```python
from build123d import *

# Parameters (mm, degrees)
SKETCH1_W           = 42
SKETCH1_H           = 42
BOSS_EXTRUDE1_DEPTH = 2
CUT_EXTRUDE1_DEPTH  = 10
SKETCH3_R           = 5
CUT_EXTRUDE2_DEPTH  = 10
SKETCH4_R           = 2
CUT_EXTRUDE3_DEPTH  = 10
SKETCH5_W           = 7
SKETCH5_H           = 10
CUT_EXTRUDE4_DEPTH  = 4


with BuildPart() as part:
    # Sketch1 → Boss-Extrude1 (new body)
    with BuildSketch(Plane(origin=(0, 0, 0), x_dir=(1, 0, 0), z_dir=(0, 1, 0))):
        Rectangle(SKETCH1_W, SKETCH1_H)
    extrude(amount=BOSS_EXTRUDE1_DEPTH)

    # Sketch2 → Cut-Extrude1 (cut)
    with BuildSketch(Plane(origin=(0, 2, 0), x_dir=(1, 0, 0), z_dir=(0, 1, 0))):
        Polygon((-16.050252532, 21), (-21, 21), (-21, 16.050252532), align=None)
        Polygon((21, 21), (16.050252532, 21), (21, 16.050252532), align=None)
        Polygon((21, -16.050252532), (16.050252532, -21), (21, -21), align=None)
        Polygon((-16.050252532, -21), (-21, -16.050252532), (-21, -21), align=None)
    extrude(amount=-CUT_EXTRUDE1_DEPTH, mode=Mode.SUBTRACT)

    # Sketch3 → Cut-Extrude2 (cut)
    with BuildSketch(Plane(origin=(0, 2, 0), x_dir=(1, 0, 0), z_dir=(0, 1, 0))):
        with Locations(Location((0, 0, 0), (0, 0, 270))):
            Circle(SKETCH3_R)
    extrude(amount=-CUT_EXTRUDE2_DEPTH, mode=Mode.SUBTRACT)

    # Sketch4 → Cut-Extrude3 (cut)
    with BuildSketch(Plane.XZ):
        with Locations(Location((6.5, 15.5, 0), (0, 0, 270))):
            Circle(SKETCH4_R)
        with Locations(Location((-6.5, -15.5, 0), (0, 0, 270))):
            Circle(SKETCH4_R)
    extrude(amount=-CUT_EXTRUDE3_DEPTH, mode=Mode.SUBTRACT)

    # Sketch5 → Cut-Extrude4 (cut)
    with BuildSketch(Plane.XZ):
        with Locations((0, -16)):
            Rectangle(SKETCH5_W, SKETCH5_H)
        with Locations((0, 16)):
            Rectangle(SKETCH5_W, SKETCH5_H)
    extrude(amount=-CUT_EXTRUDE4_DEPTH, mode=Mode.SUBTRACT)


solid = part.part
```
For this review, take the finished solid that the model builds, in its own axes (mm). A direction names the side the tool comes from. Round coordinates to 2 decimals unless told otherwise and drop trailing zeros. Loops run counter-clockwise (first coordinate to the right, second up) from the corner with the lowest first, then second, coordinate; pieces in that order, holes last.
Q1. Add section D-D on z = 15.5. Write out the cut boundary in (x, y).
Result sheet:
outline: (-21, 0) - (-3.5, 0) - (-3.5, 2) - (-21, 2) - close; (3.5, 0) - (4.5, 0) - (4.5, 2) - (3.5, 2) - close; (8.5, 0) - (21, 0) - (21, 2) - (8.5, 2) - close
Q2. Add section C-C on y = 1.15. Write out the cut boundary in (x, z).
Result sheet:
outline: (-21, -16.05) - (-16.05, -21) - (-3.5, -21) - (-3.5, -11) - (3.5, -11) - (3.5, -21) - (16.05, -21) - (21, -16.05) - (21, 16.05) - (16.05, 21) - (3.5, 21) - (3.5, 11) - (-3.5, 11) - (-3.5, 21) - (-16.05, 21) - (-21, 16.05) - close; hole circle Ø4 at (-6.5, -15.5); hole circle Ø10 at (0, 0); hole circle Ø4 at (6.5, 15.5)
Q3. Mouldability with a two-part tool opening along Z and no side actions: class faces 1 (the face through (4, 2, 4)), 2 (the face through (-10, 1, -21)), 3 (the face through (-4.88, 1.01, -1.08)) as +Z half, -Z half, draft (parallel to the pull), parting line (faces both ways), or undercut.
Result sheet:
face 1: draft
face 2: -Z half
face 3: undercut
Q4. Machinability: for faces 4 (the face through (3.5, 1, 16)), 5 (the face through (18.49, 1.01, -18.56)), 6 (the face through (-3.5, 1, -16)), which of the approach directions +Z, -Z, +X, -X, +Y, -Y give a long, thin tool a straight path to every point of the face, cutting with its end or side? Answer none if there is none.
Result sheet:
face 4: +Z, +Y, -Y
face 5: -Z, +X, +Y, -Y
face 6: -Z, +Y, -Y
Q5. To check wall thickness, follow line 1 along X through (y, z) = (1.15, -15.5); line 2 along X through (y, z) = (0.55, 15.5); line 3 along X through (y, z) = (0.8, -12). State the ranges of each line that lie inside material, in increasing order.
Result sheet:
line 1: x = -21 to -8.5, -4.5 to -3.5, 3.5 to 21
line 2: x = -21 to -3.5, 3.5 to 4.5, 8.5 to 21
line 3: x = -21 to -3.5, 3.5 to 21
Q6. Insertion check: pin 1 Ø0.6 at (x, y) = (1.5, 1) entering from +Z; pin 2 Ø1 at (x, y) = (1, 1.5) entering from -Z; pin 3 Ø2.5 at (x, z) = (-6.5, -15.5) entering from +Y; pin 4 Ø0.6 at (y, z) = (1, -18) entering from +X. Each pin has a flat end and moves straight along its axis. Give the tip position at first contact, or say it passes through.
Result sheet:
pin 1: stops at z = 11
pin 2: stops at z = -11
pin 3: passes through
pin 4: stops at x = 19.35
Q7. Add section A-A on x = 0. Write out the cut boundary in (y, z), plus the area to 3 significant figures.
Result sheet:
outline: (0, -11) - (2, -11) - (2, -5) - (0, -5) - close; (0, 5) - (2, 5) - (2, 11) - (0, 11) - close
area: 24.0 mm2
Q8. Add section B-B on z = 0. Write out the cut boundary in (x, y), plus the area to 3 significant figures.
Result sheet:
outline: (-21, 0) - (-5, 0) - (-5, 2) - (-21, 2) - close; (5, 0) - (21, 0) - (21, 2) - (5, 2) - close
area: 64.0 mm2
